Part print with two shaded views. Sizes in mm from the minimum x, y, z corner. A direction names the side the tool comes from. Give positions to 0.01 mm unless a question says otherwise; leave off trailing zeros. Write each loop counter-clockwise with the first axis right and the second up, starting at its lowest first coordinate (ties: lowest second). Pieces come first, ordered by that corner, then holes. Notation, with made-up numbers: (63, 89.25) - (101, 89.25) arc R24 ccw to (101, 128.25) - close; hole circle Ø2 at (0, 5.25). An arc over 180 degrees is marked (long way). One line per item, written item: value. Start each with the question number.
(1) Mould opens along Z. For the marked faces 1, 2 and 3 say: pulls with the +Z half, pulls with the -Z half, needs draft (parallel to the pull), parting line crosses it, or undercut.
(2) Drop flat-ended pins along their axis: P1, Ø12, axis at x = 7.5, y = 36, coming from the +Z side; P2, Ø7.5, axis at x = 8, y = 60.5, coming from the +Z side; P3, Ø6, axis at x = 19, z = 33.5, coming from the +Y side. Give the stop position or say it passes through.
(3) Cut at B-B, the plane y = 82.5. List the corners of the cut face in (x, z) (1 decimal).
(4) 3-axis set-ups, long thin cutter, end or side, ignore diameter. For the marked faces 4, 5 and 6: which of +Z, -Z, +X, -X, +Y, -Y reach the whole face in a straight line?
(5) Probe L1, parallel to Z at x = 21.5, y = 13; L2, parallel to Z at x = 8, y = 57; L3, parallel to X at y = 16.5, z = 5. List the from-to ranges inside material, lowest first.
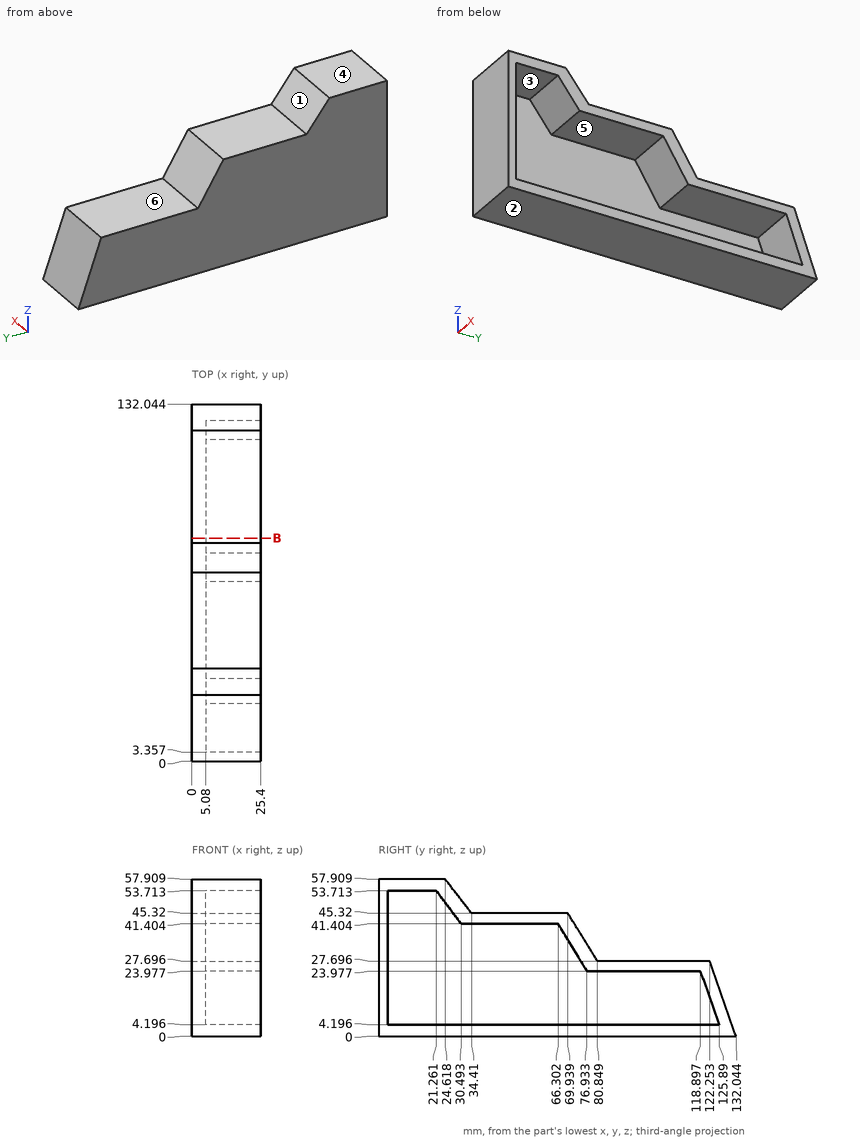
Answers follow:
1. face 1: pulls with the +Z half
1. face 2: pulls with the -Z half
1. face 3: undercut
2. P1: stops at z = 50.99
2. P2: stops at z = 45.32
2. P3: stops at y = 79.11
3. outline: (0, 0) - (25.4, 0) - (25.4, 4.2) - (5.1, 4.2) - (5.1, 24) - (25.4, 24) - (25.4, 27.7) - (0, 27.7) - close
4. face 4: +Z, +X, -X, +Y, -Y
4. face 5: +X
4. face 6: +Z, +X, -X, +Y
5. L1: z = 0 to 4.2, 53.71 to 57.91
5. L2: z = 0 to 4.2, 41.4 to 45.32
5. L3: x = 0 to 5.08
